from build123d import *

# Parameters (mm, degrees)
SKETCH11_W                               = 76.2
SKETCH11_H                               = 25.4
SKETCH11_W_2                             = 70.104
SKETCH11_H_2                             = 19.304
RECTANGULAR_TUBE_1_5_X_3_X_125_1_DEPTH   = 241.3
CBORE_FOR_1_2_HEX_HEAD_BOLT1_D           = 13.49248
CBORE_FOR_1_2_HEX_HEAD_BOLT1_CBORE_D     = 28.575
CBORE_FOR_1_2_HEX_HEAD_BOLT1_CBORE_DEPTH = 3.175
F_1_4_CLEARANCE_HOLE1_D                  = 6.7564


with BuildPart() as part:
    # Sketch11 → Rectangular tube 1.5 X 3 X .125(1) (new body)
    with BuildSketch(Plane.ZY.offset(-120.65)):
        Rectangle(SKETCH11_W, SKETCH11_H)
        Rectangle(SKETCH11_W_2, SKETCH11_H_2, mode=Mode.SUBTRACT)
    extrude(amount=RECTANGULAR_TUBE_1_5_X_3_X_125_1_DEPTH)

    # CBORE for 1/2 Hex Head Bolt1 (through all)
    with Locations(Plane(origin=(0, -12.7, 0), x_dir=(-1, 0, 0), z_dir=(0, -1, 0))):
        with Locations((50.8, 0), (-50.8, 0)):
            CounterBoreHole(CBORE_FOR_1_2_HEX_HEAD_BOLT1_D / 2, CBORE_FOR_1_2_HEX_HEAD_BOLT1_CBORE_D / 2, CBORE_FOR_1_2_HEX_HEAD_BOLT1_CBORE_DEPTH)

    # 1/4 Clearance Hole1 (through all)
    with Locations(Plane(origin=(0, -12.7, 0), x_dir=(-1, 0, 0), z_dir=(0, -1, 0))):
        with Locations((107.95, -25.4), (107.95, 25.4), (-107.95, 25.4), (-107.95, -25.4)):
            Hole(F_1_4_CLEARANCE_HOLE1_D / 2)


solid = part.part
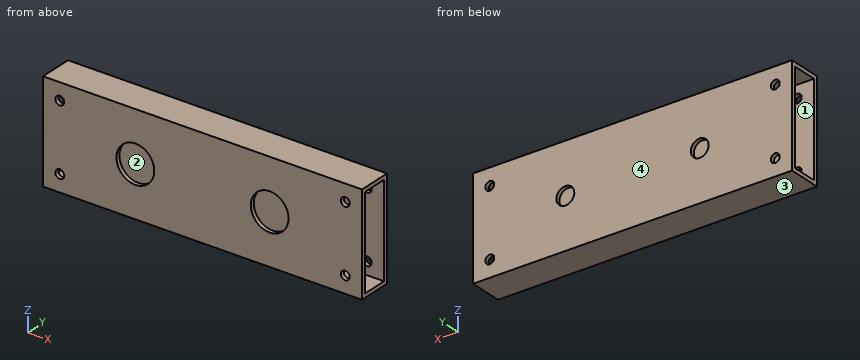
Read the model definition and answer for the solid it produces. Units are mm, in the model's axes. Face numbers are marked on the shaded views. Give positions to 0.01 mm unless a question says otherwise; leave off trailing zeros. Write each loop counter-clockwise with the first axis right and the second up, starting at its lowest first coordinate (ties: lowest second). Pieces come first, ordered by that corner, then holes. Notation, with made-up numbers: (88.5, -16.75) - (102.5, -16.75) arc R19 cw to (102.5, -5.75) - close; hole circle Ø11 at (55.5, 49.5). An arc over 180 degrees is marked (long way). Use CSV: the item, a comma, the result in double quotes. Start each with the question number.
Item 1: The part is cut by section A-A, the plane z = -17. Give the vertices of the cut face in (x, y).
Item 2: Consider line 1 (Z direction, x = -107.95, y = 11.9); line 2 (X direction, y = -11.8, z = -25.4); line 3 (Y direction, x = 30.5, z = -4). Determine where each line is inside the solid, lowest interval first.
Item 3: A flat-ended cylindrical pin translates along its axis: P1, Ø23, axis at x = 50.8, z = 0, coming from the -Y side. Find the tip coordinate at first contact, or state that the pin passes through.
Item 4: The mould has two halves that part along Z. Classify the marked faces 1, 2, 3 and 4: pulls with the +Z half, pulls with the -Z half, needs draft (parallel to the pull), parting line crosses it, or undercut.
Item 5: The part is cut by section B-B, the plane y = -2. Give the vertices of the cut face in (x, z).
Item 6: The part is cut by section C-C, the plane x = 50.8. Give the vertices of the cut face in (y, z).
Item 7: The part is cut by section D-D, the plane x = -2. Give the vertices of the cut face in (y, z).
Taken from the geometry:
1,outline,"(-120.65, -12.7) - (120.65, -12.7) - (120.65, -9.65) - (-120.65, -9.65) - close; (-120.65, 9.65) - (120.65, 9.65) - (120.65, 12.7) - (-120.65, 12.7) - close"
2,line 1,"-38.1 to -28.78, -22.02 to 22.02, 28.78 to 38.1"
2,line 2,"-120.65 to -111.33, -104.57 to 104.57, 111.33 to 120.65"
2,line 3,"-12.7 to -9.65, 9.65 to 12.7"
3,P1,"y = 9.65"
4,face 1,"undercut"
4,face 2,"undercut"
4,face 3,"pulls with the -Z half"
4,face 4,"needs draft"
5,outline,"(-120.65, -38.1) - (120.65, -38.1) - (120.65, -35.05) - (-120.65, -35.05) - close; (-120.65, 35.05) - (120.65, 35.05) - (120.65, 38.1) - (-120.65, 38.1) - close"
6,outline,"(-12.7, -38.1) - (12.7, -38.1) - (12.7, -6.75) - (9.65, -6.75) - (9.65, -35.05) - (-9.65, -35.05) - (-9.65, -14.29) - (-12.7, -14.29) - close; (-12.7, 14.29) - (-9.65, 14.29) - (-9.65, 35.05) - (9.65, 35.05) - (9.65, 6.75) - (12.7, 6.75) - (12.7, 38.1) - (-12.7, 38.1) - close"
7,outline,"(-12.7, -38.1) - (12.7, -38.1) - (12.7, 38.1) - (-12.7, 38.1) - close; hole (-9.65, -35.05) - (9.65, -35.05) - (9.65, 35.05) - (-9.65, 35.05) - close"
